Read the model definition and answer for the solid it produces. Units are mm, in the model's axes. A direction names the side the tool comes from. Give positions to 0.01 mm unless a question says otherwise; leave off trailing zeros. Write each loop counter-clockwise with the first axis right and the second up, starting at its lowest first coordinate (ties: lowest second). Pieces come first, ordered by that corner, then holes. Notation, with made-up numbers: (-5, -38.75) - (23, -38.75) arc R22 ccw to (23, -13.75) - close; hole circle Ø2 at (17.5, -22). An arc over 180 degrees is marked (long way). Answer as CSV lines item,"result".
```python
from build123d import *

# Parameters (mm, degrees)
SKETCH1_W           = 515.5
SKETCH1_H           = 25.4
SKETCH1_R           = 3.175
BOSS_EXTRUDE1_DEPTH = 25.4
CUT_EXTRUDE1_REACH  = 518.75
SKETCH2_W           = 19.05
SKETCH2_H           = 19.05
SKETCH4_W           = 25.4
SKETCH4_H           = 19.05
CUT_EXTRUDE2_DEPTH  = 38.1
FILLET1_R           = 20


with BuildPart() as part:
    # Sketch1 → Boss-Extrude1 (new body)
    with BuildSketch(Plane(origin=(0, 0, 0), x_dir=(1, 0, 0), z_dir=(0, 1, 0))):
        with Locations((257.75, -12.7)):
            Rectangle(SKETCH1_W, SKETCH1_H)
        with Locations(Location((257.75, -12.7, 0), (0, 0, 270))):
            Circle(SKETCH1_R, mode=Mode.SUBTRACT)
        with Locations(Location((20.76, -12.7, 0), (0, 0, 270))):
            Circle(SKETCH1_R, mode=Mode.SUBTRACT)
        with Locations(Location((494.74, -12.7, 0), (0, 0, 90))):
            Circle(SKETCH1_R, mode=Mode.SUBTRACT)
    extrude(amount=BOSS_EXTRUDE1_DEPTH)

    # Cut-Extrude1: up to this face of the body (flat: up to its plane)
    cut_extrude1_end = Plane(part.part.faces().sort_by_distance((515.5, 12.7, 12.7))[0])
    # Sketch2 → Cut-Extrude1 (cut, up to the picked face)
    with BuildSketch(Plane.ZY, mode=Mode.PRIVATE) as cut_extrude1_sk1:
        with Locations((12.7, 12.7)):
            Rectangle(SKETCH2_W, SKETCH2_H)
    cut_extrude1_tool1 = split(extrude(cut_extrude1_sk1.sketch, amount=-CUT_EXTRUDE1_REACH, mode=Mode.PRIVATE), bisect_by=cut_extrude1_end, keep=Keep.BOTH, mode=Mode.PRIVATE)
    add(cut_extrude1_tool1.solids().sort_by(Axis((0, 12.7, 12.7), (1, 0, 0)))[0], mode=Mode.SUBTRACT)

    # Sketch4 → Cut-Extrude2 (cut)
    with BuildSketch(Plane.ZY):
        with Locations((12.7, 12.7)):
            Rectangle(SKETCH4_W, SKETCH4_H)
    cut_extrude2 = extrude(amount=-CUT_EXTRUDE2_DEPTH, mode=Mode.SUBTRACT)

    # Mirror1: Cut-Extrude2 across plane
    add(cut_extrude2.mirror(Plane.ZY.offset(-257.75)), mode=Mode.SUBTRACT)

    # Fillet1
    # the kernel refuses this fillet: 20 mm, written as the material it takes off along each edge
    with BuildSketch(Plane(origin=(515.5, -50, 0), x_dir=(-1, 0, 0), z_dir=(0, 1, 0)), Plane(origin=(515.5, -27.775, 0), x_dir=(-1, 0, 0), z_dir=(0, 1, 0)), Plane(origin=(0, -27.775, 25.4), x_dir=(1, 0, 0), z_dir=(0, 1, 0))) as fillet1_piece_1:
        with BuildLine():
            CenterArc((FILLET1_R, FILLET1_R), FILLET1_R, 180, 90)
            Line((0, FILLET1_R), (0, 0))
            Line((0, 0), (FILLET1_R, 0))
        make_face()
    extrude(amount=103.175, mode=Mode.SUBTRACT)
    with BuildSketch(Plane(origin=(515.5, -50, 25.4), x_dir=(-1, 0, 0), z_dir=(0, 1, 0)), Plane(origin=(515.5, -27.775, 25.4), x_dir=(-1, 0, 0), z_dir=(0, 1, 0)), Plane(origin=(0, -50, 25.4), x_dir=(0, 0, -1), z_dir=(0, 1, 0)), Plane(origin=(0, -50, 0), x_dir=(1, 0, 0), z_dir=(0, 1, 0)), Plane(origin=(0, -27.775, 0), x_dir=(1, 0, 0), z_dir=(0, 1, 0))) as fillet1_piece_2:
        with BuildLine():
            CenterArc((FILLET1_R, -FILLET1_R), FILLET1_R, 90, 90)
            Line((0, -FILLET1_R), (0, 0))
            Line((0, 0), (FILLET1_R, 0))
        make_face()
    extrude(amount=103.175, mode=Mode.SUBTRACT)


solid = part.part
```
(1) For faces 4 (the flat face through (255, 13, 3.175)), 5 (the cylindrical face through (8.593, 23.79, 21.828)), determine the directions among +Z, -Z, +X, -X, +Y, -Y from which every point of the face is accessible in a straight line to the end or side of a thin tool.
Worked out:
face 4,"+X, -X"
face 5,"+Z, -X, +Y, -Y"
(2) A cutting plane is placed at B-B (x = 345). Write down the section's boundary in (y, z) (3 decimals).
Worked out:
outline,"(0, 0) - (25.4, 0) - (25.4, 25.4) - (0, 25.4) - close; hole (3.175, 3.175) - (22.225, 3.175) - (22.225, 22.225) - (3.175, 22.225) - close"
(3) Each of these flat-tipped pins is pushed along its axis until it touches: P1, Ø1, axis at y = 15.5, z = 1, coming from the -X side; P2, Ø3.5, axis at y = 11, z = 24.5, coming from the +X side; P3, Ø7.5, axis at x = 240, z = 8, coming from the -Y side; P4, Ø2, axis at y = 3.5, z = 20.5, coming from the +X side. Where does it stop, or does it pass through?
Worked out:
P1,"stops at x = 38.1"
P2,"stops at x = 477.4"
P3,"stops at y = 0"
P4,"stops at x = 509.63"
(4) The mould has two halves that part along Z. Classify faces 1 (the flat face through (254, 0, 13)), 2 (the flat face through (254, 3.175, 13)), 3 (the cylindrical face through (506.631, 23.79, 22.017)): +Z half, -Z half, draft (parallel to the pull), parting line (faces both ways), or undercut.
Worked out:
face 1,"draft"
face 2,"undercut"
face 3,"+Z half"
(5) Find the intervals of material crossed by L1, parallel to Z at x = 20.76, y = 24.65 (3 decimals); L2, parallel to Z at x = 403.5, y = 17.5 (3 decimals), in increasing order.
Worked out:
L1,"z = 0 to 9.525, 15.875 to 25.4"
L2,"z = 0 to 3.175, 22.225 to 25.4"
(6) A cutting plane is placed at A-A (y = 10.25). Write down the section's boundary in (x, z) (3 decimals).
Worked out:
outline,"(38.1, 0) - (477.4, 0) - (477.4, 3.175) - (38.1, 3.175) - close; (38.1, 22.225) - (477.4, 22.225) - (477.4, 25.4) - (38.1, 25.4) - close"
